```python
from build123d import *

# Parameters (mm, degrees)
SKETCH_1_R          = 1.9
EXTRUDE_1_DEPTH     = 72
SKETCH_2_R          = 2.25
CUT_EXTRUDE_1_DEPTH = 2.1


with BuildPart() as part:
    # 草图1 → 凸台-拉伸1 (new body)
    with BuildSketch(Plane(origin=(0, 0, 0), x_dir=(0, 0, -1), z_dir=(1, 0, 0))):
        with BuildLine():
            Line((0, 0), (19, 0))
            Line((19, 0), (19, -1.1))
            Line((19, -1.1), (0, -1.1))
            Line((0, -1.1), (-3, -1.1))
            ThreePointArc((-3, -1.1), (-4.284523258, 4.611088342), (-0.678362647, 0))
            Line((-0.678362647, 0), (0, 0))
        make_face()
        with Locations((-3, 1.9)):
            Circle(SKETCH_1_R, mode=Mode.SUBTRACT)
    extrude(amount=EXTRUDE_1_DEPTH)

    # 草图2 → 切除-拉伸1 (cut, through all)
    with BuildSketch(Plane(origin=(0, 0, 0), x_dir=(1, 0, 0), z_dir=(0, 1, 0))):
        with Locations((8.15, 10.85)):
            Circle(SKETCH_2_R)
        with Locations((63.85, 10.85)):
            Circle(SKETCH_2_R)
    extrude(amount=-CUT_EXTRUDE_1_DEPTH, mode=Mode.SUBTRACT)


solid = part.part
```
For this review, take the finished solid that the model builds, in its own axes (mm). Give positions to 0.01 mm unless a question says otherwise; leave off trailing zeros. Write each loop counter-clockwise with the first axis right and the second up, starting at its lowest first coordinate (ties: lowest second). Pieces come first, ordered by that corner, then holes.
Item 1: Wall thickness on probe 1 along X at (y, z) = (-0.8, -10.85); probe 2 along Y at (x, z) = (20, 3); probe 3 along Z at (x, y) = (65.5, 0.4): over which ranges is each line inside the solid? List them lowest first.
Item 2: The part is to be moulded in two halves that separate along Z. For faces 1 (the face through (0, -0.5, -3.8)), 2 (the face through (65.996, -0.542, -11.526)), 3 (the face through (35.496, 1.172, 1.245)), say which applies: +Z half, -Z half, draft (parallel to the pull), parting line (faces both ways), or undercut.
Item 3: Take a section at D-D (x = 21). Give the boundary of the cut face in (y, z), and give its area (3 significant figures).
Item 4: Take a section at B-B (y = 1.9). Give the boundary of the cut face in (x, z).
Item 5: Take a section at A-A (z = -10.85). Give the boundary of the cut face in (x, y), and give its area (3 significant figures).
Item 6: Take a section at C-C (x = 63.85). Give the boundary of the cut face in (y, z).
Item 7: Insertion check: P1, Ø10, axis at x = 48.5, z = -8, coming from the +Y side; P2, Ø1, axis at x = 31.5, y = 3.5, coming from the +Z side; P3, Ø3, axis at x = 55.5, y = 3, coming from the -Z side. Each pin has a flat end and moves straight along its axis. Give the tip position at first contact, or say it passes through.
Established:
1. probe 1: x = 0 to 5.9, 10.4 to 61.6, 66.1 to 72
1. probe 2: y = -1.1 to 0, 3.8 to 4.9
1. probe 3: z = 0.4 to 1.83, 4.17 to 5.6
2. face 1: draft
2. face 2: undercut
2. face 3: undercut
3. outline: (-1.1, -19) - (0, -19) - (0, 0.68) arc R3 ccw (long way) to (-1.1, 3) - close; hole circle Ø3.8 at (1.9, 3)
3. area: 39.4 mm2
4. outline: (0, 0) - (72, 0) - (72, 1.1) - (0, 1.1) - close; (0, 4.9) - (72, 4.9) - (72, 6) - (0, 6) - close
5. outline: (0, -1.1) - (5.9, -1.1) - (5.9, 0) - (0, 0) - close; (10.4, -1.1) - (61.6, -1.1) - (61.6, 0) - (10.4, 0) - close; (66.1, -1.1) - (72, -1.1) - (72, 0) - (66.1, 0) - close
5. area: 69.3 mm2
6. outline: (-1.1, -19) - (0, -19) - (0, -13.1) - (-1.1, -13.1) - close; (-1.1, -8.6) - (0, -8.6) - (0, 0.68) arc R3 ccw (long way) to (-1.1, 3) - close; hole circle Ø3.8 at (1.9, 3)
7. P1: stops at y = 0
7. P2: stops at z = 5.79
7. P3: stops at z = 0
